```python
from build123d import *

# Parameters (mm, degrees)
EXTRUDE_1_DEPTH         = 3
SKETCH_3_R              = 7.6
SKETCH_3_R_2            = 9.5
SKETCH_3_R_3            = 1.55
CUT_EXTRUDE_1_DEPTH     = 112.843640856
EXTRUDE_6_DEPTH         = 3
SKETCH_10_R             = 1.55
CUT_EXTRUDE_3_DEPTH     = 124.991771172
CUT_EXTRUDE_6_DEPTH     = 124.991771172
EXTRUDE_7_DEPTH         = 3
CUT_EXTRUDE_7_DEPTH     = 124.991771172
SKETCH_18_W             = 9.7
SKETCH_18_H             = 35
CUT_EXTRUDE_9_DEPTH     = 124.991771172
SKETCH_19_R             = 1.55
CUT_EXTRUDE_10_DEPTH    = 124.991771172
SKETCH_20_W             = 61.573881036
SKETCH_20_H             = 3.2
SKETCH_20_W_2           = 79.598608315
SKETCH_20_H_2           = 1.2
EXTRUDE_8_DEPTH         = 3
EXTRUDE_START           = -3
EXTRUDE_9_DEPTH         = 3
EXTRUDE_11_DEPTH        = 3
SKETCH_25_R             = 9.5
EXTRUDE_12_DEPTH        = 3
SKETCH_26_R             = 9.5
CUT_EXTRUDE_11_DEPTH    = 124.991771172
EXTRUDE_13_DEPTH        = 3
CUT_EXTRUDE_12_DEPTH    = 3
SKETCH_29_W             = 5.5
SKETCH_29_H             = 32
EXTRUDE_14_DEPTH        = 3
SKETCH_32_W             = 9.716106013
SKETCH_32_H             = 6
CUT_EXTRUDE_13_DEPTH    = 124.991771172
CUT_EXTRUDE_16_DEPTH    = 3
SKETCH_35_W             = 2.5
SKETCH_35_H             = 44.4
EXTRUDE_15_DEPTH        = 3
SKETCH_36_R             = 1.55
CUT_EXTRUDE_14794_DEPTH = 3
EXTRUDE_16_DEPTH        = 3
SKETCH_38_R             = 2.75
CUT_EXTRUDE_L_DEPTH     = 121.232106085
SKETCH_41_R             = 1.55
EXTRUDE_17_DEPTH        = 3
CUT_EXTRUDE_17_DEPTH    = 121.232106085


# Read off the part's stored shape, not the designer's step: 高级异型孔1
with BuildPart() as part:
    # 草图1 → 凸台-拉伸1 (new body)
    with BuildSketch(Plane(origin=(0, 0, 0), x_dir=(0, 0, -1), z_dir=(1, 0, 0))):
        Polygon((0, -50), (18.610302832, -39.45792997), (18.610302832, 40), (58.496702951, 40), (58.496702951, 0), (100, 0), (100, -50), align=None)
    extrude(amount=EXTRUDE_1_DEPTH)

    # 草图3 → 切除-拉伸1 (cut, through all)
    with BuildSketch(Plane.ZY):
        with Locations((-74, -24.961577338)):
            Circle(SKETCH_3_R)
        with Locations((-34.176393222, 0)):
            Circle(SKETCH_3_R_2)
        with Locations((-74, -7.461577338)):
            Circle(SKETCH_3_R_3)
        with Locations((-56.5, -24.961577338)):
            Circle(SKETCH_3_R_3)
        with Locations((-74, -42.461577338)):
            Circle(SKETCH_3_R_3)
        with Locations((-91.5, -24.961577338)):
            Circle(SKETCH_3_R_3)
    extrude(amount=-CUT_EXTRUDE_1_DEPTH, mode=Mode.SUBTRACT)

    # 草图6 → 凸台-拉伸6 (add)
    with BuildSketch(Plane.ZY):
        with BuildLine():
            Line((-102.983893987, -45.2), (-110.983893987, -45.2))
            Line((-110.983893987, -45.2), (-111, -50))
            Line((-111, -50), (-100, -50))
            Line((-100, -50), (-100, 0))
            Line((-100, 0), (-110.983893987, 0))
            Line((-110.983893987, 0), (-110.983893987, -6.8))
            Line((-110.983893987, -6.8), (-102.983893987, -6.8))
            ThreePointArc((-102.983893987, -6.8), (-101.283893987, -8.5), (-102.983893987, -10.2))
            Line((-102.983893987, -10.2), (-110.983893987, -10.2))
            Line((-110.983893987, -10.2), (-110.983893987, -41.8))
            Line((-110.983893987, -41.8), (-102.983893987, -41.8))
            ThreePointArc((-102.983893987, -41.8), (-101.283893987, -43.5), (-102.983893987, -45.2))
        make_face()
        with BuildLine():
            Line((-15.00347976, -50), (-34.686448159, -50))
            ThreePointArc((-34.686448159, -50), (-33.16855591, -50.235967767), (-31.793933119, -50.921598751))
            Line((-31.793933119, -50.921598751), (-26.580472983, -54.619128968))
            ThreePointArc((-26.580472983, -54.619128968), (-25.755699309, -55.030507559), (-24.844963959, -55.172088219))
            ThreePointArc((-24.844963959, -55.172088219), (-23.93422861, -55.030507559), (-23.109454935, -54.619128968))
            Line((-23.109454935, -54.619128968), (-17.8959948, -50.921598751))
            ThreePointArc((-17.8959948, -50.921598751), (-16.521372009, -50.235967767), (-15.00347976, -50))
        make_face()
    extrude(amount=-EXTRUDE_6_DEPTH)

    # 草图10 → 切除-拉伸3 (cut, through all)
    with BuildSketch(Plane.ZY):
        with Locations((-105.983893987, -15.2)):
            Circle(SKETCH_10_R)
        with Locations((-105.983893987, -36.8)):
            Circle(SKETCH_10_R)
    extrude(amount=-CUT_EXTRUDE_3_DEPTH, mode=Mode.SUBTRACT)

    # 草图14 → 切除-拉伸6 (cut, through all)
    with BuildSketch(Plane(origin=(3, 0, 0), x_dir=(0, 0, -1), z_dir=(1, 0, 0))):
        with BuildLine():
            Line((58.496702951, 0), (58.496702951, 40))
            Line((58.496702951, 40), (18.610302832, 40))
            Line((18.610302832, 40), (18.610302832, 18.686206016))
            ThreePointArc((18.610302832, 18.686206016), (44.493983197, 22.023278649), (58.496702951, 0))
        make_face()
    extrude(amount=-CUT_EXTRUDE_6_DEPTH, mode=Mode.SUBTRACT)

    # 草图15 → 凸台-拉伸7 (add)
    with BuildSketch(Plane(origin=(3, 0, 0), x_dir=(0, 0, -1), z_dir=(1, 0, 0))):
        with BuildLine():
            Line((18.610302832, 18.686206016), (18.610302832, -18.686206016))
            ThreePointArc((18.610302832, -18.686206016), (9.856083494, 0), (18.610302832, 18.686206016))
        make_face()
    extrude(amount=-EXTRUDE_7_DEPTH)

    # 草图16 → 切除-拉伸7 (cut, through all)
    with BuildSketch(Plane(origin=(3, 0, 0), x_dir=(0, 0, -1), z_dir=(1, 0, 0))):
        with BuildLine():
            Line((18.610302832, -18.686206016), (18.610302832, 0))
            ThreePointArc((18.610302832, 0), (34.176393222, 15.56609039), (49.742483613, 0))
            Line((49.742483613, 0), (58.496702951, 0))
            ThreePointArc((58.496702951, 0), (23.858803248, 22.023278649), (18.610302832, -18.686206016))
        make_face()
    extrude(amount=-CUT_EXTRUDE_7_DEPTH, mode=Mode.SUBTRACT)

    # 草图18 → 切除-拉伸9 (cut, through all)
    with BuildSketch(Plane.ZY):
        with Locations((-106.133893987, -26)):
            Rectangle(SKETCH_18_W, SKETCH_18_H)
    extrude(amount=-CUT_EXTRUDE_9_DEPTH, mode=Mode.SUBTRACT)

    # 草图19 → 切除-拉伸10 (cut, through all)
    with BuildSketch(Plane.ZY):
        with Locations((-105.983893987, -1.8)):
            Circle(SKETCH_19_R)
        with Locations((-105.993932098, -48.2)):
            Circle(SKETCH_19_R)
    extrude(amount=-CUT_EXTRUDE_10_DEPTH, mode=Mode.SUBTRACT)

    # 草图20 → 凸台-拉伸8 (add)
    with BuildSketch(Plane.ZY):
        with Locations((-80.196953469, 1.6)):
            Rectangle(SKETCH_20_W, SKETCH_20_H)
        with Locations((-71.200695842, -50.6)):
            Rectangle(SKETCH_20_W_2, SKETCH_20_H_2)
    extrude(amount=-EXTRUDE_8_DEPTH)

    # 草图22 → 凸台-拉伸9 (add)
    with BuildSketch(Plane.ZY.offset(EXTRUDE_START)):
        with BuildLine():
            Line((-18.610302832, 0), (-18.610302832, 25))
            Line((-18.610302832, 25), (-41.044918155, 13.968769999))
            ThreePointArc((-41.044918155, 13.968769999), (-25.948784515, 13.213993529), (-18.610302832, 0))
        make_face()
    extrude(amount=EXTRUDE_9_DEPTH)

    # 草图24 → 凸台-拉伸11 (add)
    with BuildSketch(Plane.ZY):
        Polygon((-18.610302832, 25), (-70.983893987, 3.2), (-49.410012951, 3.2), align=None)
    extrude(amount=-EXTRUDE_11_DEPTH)

    # 草图25 → 凸台-拉伸12 (add, through all)
    with BuildSketch(Plane(origin=(3, 0, 0), x_dir=(0, 0, -1), z_dir=(1, 0, 0))):
        with Locations((34.176393222, 0)):
            Circle(SKETCH_25_R)
    extrude(amount=-EXTRUDE_12_DEPTH)

    # 草图26 → 切除-拉伸11 (cut, through all)
    with BuildSketch(Plane(origin=(3, 0, 0), x_dir=(0, 0, -1), z_dir=(1, 0, 0))):
        with Locations((29.059828781, -15.2)):
            Circle(SKETCH_26_R)
    extrude(amount=-CUT_EXTRUDE_11_DEPTH, mode=Mode.SUBTRACT)

    # 草图27 → 凸台-拉伸13 (add)
    with BuildSketch(Plane.ZY):
        Polygon((-18.610302832, -10.2), (-13.610302832, -15.2), (-18.610302832, -20.2), align=None)
    extrude(amount=-EXTRUDE_13_DEPTH)

    # 草图28 → 切除-拉伸12 (cut)
    with BuildSketch(Plane.ZY):
        Polygon((-110.983893987, 3.2), (-101.283893987, 3.2), (-70.983893987, 3.2), (-95.008477086, -6.8), (-101.283893987, -6.8), (-101.283893987, -45.2), (-110.983893987, -45.2), align=None)
    extrude(amount=-CUT_EXTRUDE_12_DEPTH, mode=Mode.SUBTRACT)

    # 草图29 → 凸台-拉伸14 (add)
    with BuildSketch(Plane.ZY):
        with Locations((-104.033893987, -27.7)):
            Rectangle(SKETCH_29_W, SKETCH_29_H)
    extrude(amount=-EXTRUDE_14_DEPTH)

    # 草图32 → 切除-拉伸13 (cut, through all)
    with BuildSketch(Plane.ZY):
        with Locations((-106.141946993, -48.2)):
            Rectangle(SKETCH_32_W, SKETCH_32_H)
    extrude(amount=-CUT_EXTRUDE_13_DEPTH, mode=Mode.SUBTRACT)

    # 草图34 → 切除-拉伸16 (cut)
    with BuildSketch(Plane.ZY):
        Polygon((-103.783893987, -15.75), (-103.783893987, -12.55), (-106.783893987, -13.5), (-106.783893987, -14.8), align=None)
        Polygon((-106.783893987, -18), (-106.783893987, -19.3), (-103.783893987, -20.25), (-103.783893987, -17.05), align=None)
        Polygon((-106.783893987, -22.5), (-106.783893987, -23.8), (-103.783893987, -24.75), (-103.783893987, -21.55), align=None)
        Polygon((-106.783893987, -27), (-106.783893987, -28.3), (-103.783893987, -29.25), (-103.783893987, -26.05), align=None)
        Polygon((-106.783893987, -31.5), (-106.783893987, -32.8), (-103.783893987, -33.75), (-103.783893987, -30.55), align=None)
        Polygon((-106.783893987, -36), (-106.783893987, -37.3), (-103.783893987, -38.25), (-103.783893987, -35.05), align=None)
        Polygon((-106.783893987, -40.5), (-106.783893987, -41.8), (-103.783893987, -42.75), (-103.783893987, -39.55), align=None)
    extrude(amount=-CUT_EXTRUDE_16_DEPTH, mode=Mode.SUBTRACT)

    # 草图35 → 凸台-拉伸15 (add, through all)
    with BuildSketch(Plane.ZY):
        with Locations((-102.533893987, -29)):
            Rectangle(SKETCH_35_W, SKETCH_35_H)
    extrude(amount=-EXTRUDE_15_DEPTH)

    # 草图36 → Cut-Extrude 14794 (cut)
    with BuildSketch(Plane.ZY):
        with Locations((-93.783893987, -48.2)):
            Circle(SKETCH_36_R)
        with Locations(Location((-93.783893987, -12.9, 0), (0, 0, 180))):
            Circle(SKETCH_36_R)
        with Locations((-21.610302832, 20.501770791)):
            Circle(SKETCH_36_R)
        with Locations((-11.382694019, -47)):
            Circle(SKETCH_36_R)
        with Locations(Location((-54.216106013, -48.2, 0), (0, 0, 180))):
            Circle(SKETCH_36_R)
    extrude(amount=-CUT_EXTRUDE_14794_DEPTH, mode=Mode.SUBTRACT)

    # 草图37 → 凸台-拉伸16 (add)
    with BuildSketch(Plane.ZY):
        Polygon((-13.610302832, -39.45792997), (-13.610302832, -42.290250896), (-18.610302832, -39.45792997), (-18.610302832, 25), (-13.610302832, 25), align=None)
    extrude(amount=-EXTRUDE_16_DEPTH)

    # 草图38 → L型支架定位孔 (cut, through all)
    with BuildSketch(Plane(origin=(3, 0, 0), x_dir=(0, 0, -1), z_dir=(1, 0, 0))):
        with Locations((100.283893987, -38.15)):
            Circle(SKETCH_38_R)
        with Locations((93.283893987, -33.15)):
            Circle(SKETCH_38_R)
    extrude(amount=-CUT_EXTRUDE_L_DEPTH, mode=Mode.SUBTRACT)

    # 高级异型孔1 outline → 高级异型孔1 (revolve, cut)
    with BuildSketch(Plane(origin=(0, -24.961577338, -56.5), x_dir=(0, 1, 0), z_dir=(0, 0, -1))):
        Polygon((1.7, 1.6), (1.55, 1.6), (1.55, 0), (3.3, 0), align=None)
    revolve(axis=Axis((0, -24.961577338, -56.5), (1, 0, 0)), mode=Mode.SUBTRACT)

    # 草图41 → 凸台-拉伸17 (add, through all)
    with BuildSketch(Plane.ZY):
        with Locations((-21.610302832, 20.501770791)):
            Circle(SKETCH_41_R)
    extrude(amount=-EXTRUDE_17_DEPTH)

    # 草图42 → 切除-拉伸17 (cut, through all)
    with BuildSketch(Plane.ZY):
        Polygon((-95.008477086, -6.8), (-18.610302832, 20.82), (-13.610302832, 20.82), (-13.610302832, 25), (-18.610302832, 25), align=None)
    extrude(amount=-CUT_EXTRUDE_17_DEPTH, mode=Mode.SUBTRACT)


solid = part.part
```
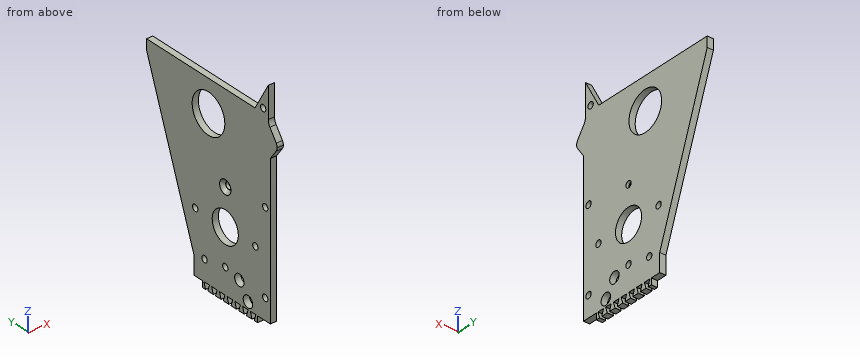
Here's how the part is built. I have some questions about the finished solid (model axes, mm). Give positions to 0.01 mm unless a question says otherwise; leave off trailing zeros. Order: outer loops, then holes, each group sorted by start corner. A loop starts at its lowest first (then second) coordinate and runs counter-clockwise, first axis right, second up. Notation, with made-up numbers: (-36, 68.25) -> (18, 68.25) arc R26 ccw to (18, 101.25) -> close; hole circle Ø5 at (28, -17). An arc over 180 degrees is marked (long way). Use CSV: the item, a comma, the result in double quotes. Start each with the question number.
Item 1: I'm going to push flat-ended pins straight in: P1, Ø0.9, axis at x = 1.5, y = -9.5, coming from the -Z side; P2, Ø1.5, axis at x = 1.5, z = -75.5, coming from the +Y side. Where does each tip first touch, or does it pass through?
Item 2: Suppose I cut it at D-D (x = 2.45). Give the number of separate pieces and of enclosed holes in the cut face, and give its area (3 significant figures).
Item 3: Suppose I cut it at A-A (z = -74). List the corners of the cut face in (x, y) for me.
Item 4: Suppose I cut it at C-C (z = -47). List the corners of the cut face in (x, y) for me, and give its area (3 significant figures).
Item 5: Suppose I cut it at B-B (y = 9). List the corners of the cut face in (x, z) for me.
Item 6: If I drill on probe 1 along Z at (x, y) = (1.95, -8); probe 2 along Y at (x, z) = (2.15, -96.5); probe 3 along Y at (x, z) = (2, -91.5), over which ranges is the centre line in solid material (lowest first)? Write a range as [from, to].
Answer block:
1,P1,"stops at z = -103.78"
1,P2,"stops at y = 0.52"
2,separate pieces,"1"
2,enclosed holes,"12"
2,area,"4,750 mm^2"
3,outline,"(0, -51.2) -> (3, -51.2) -> (3, -44.01) -> (0, -44.01) -> close; (0, -40.91) -> (3, -40.91) -> (3, -32.56) -> (0, -32.56) -> close; (0, -17.36) -> (3, -17.36) -> (3, -9.01) -> (0, -9.01) -> close; (0, -5.91) -> (3, -5.91) -> (3, 0.8) -> (0, 0.8) -> close"
4,outline,"(0, -51.2) -> (3, -51.2) -> (3, 10.56) -> (0, 10.56) -> close"
4,area,"185 mm^2"
5,outline,"(0, -51.3) -> (3, -51.3) -> (3, -13.61) -> (0, -13.61) -> close"
6,probe 1,"z = [-103.78, -75.45], [-72.55, -35.26], [-22.86, -13.61]"
6,probe 2,"y = [-51.2, -6.8]"
6,probe 3,"y = [-51.2, -35.24], [-31.06, -26.51], [-23.41, -5.53]"
